The figure shows three views and two pictorial views of one solid part (mm, origin at its lowest corner). Answer the questions. Give positions to 0.01 mm unless a question says otherwise; leave off trailing zeros. Write each loop counter-clockwise with the first axis right and the second up, starting at its lowest first coordinate (ties: lowest second). Pieces come first, ordered by that corner, then holes. Notation, with made-up numbers: (15, 24) - (51, 24) arc R23 cw to (51, 44) - close; hole circle Ø11 at (-40, 25). An arc over 180 degrees is marked (long way). Use CSV: the item, a comma, the result in double quotes. Start each with the question number.
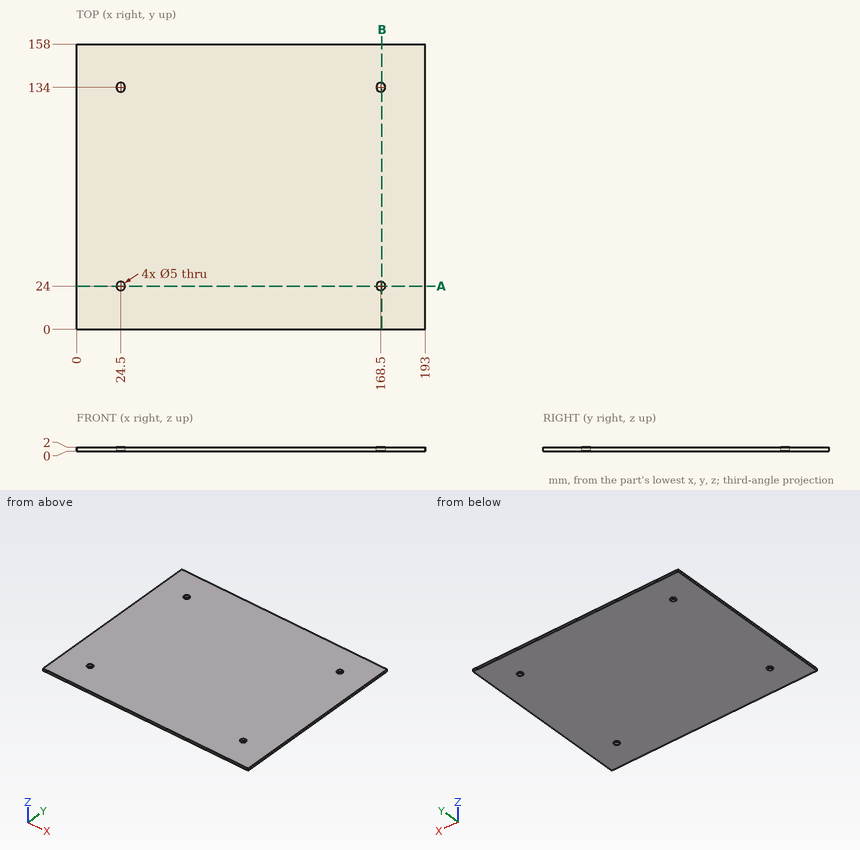
(1) Given P1, Ø8, axis at x = 168.5, y = 24, coming from the +Z side, flat-ended and moving along its own axis, determine where the tip first touches the part or whether it passes through.
(2) The part is cut by section A-A on y = 24. Write down the section's boundary in (x, z), plus the area to 3 significant figures.
(3) The part is cut by section B-B on x = 169. Write down the section's boundary in (y, z).
(4) Consider probe 1 along X at (y, z) = (134, 0.85); probe 2 along Y at (x, z) = (168.5, 1.15). Determine where each line is inside the solid, lowest interval first.
Reported:
1,P1,"z = 2"
2,outline,"(0, 0) - (22, 0) - (22, 2) - (0, 2) - close; (27, 0) - (166, 0) - (166, 2) - (27, 2) - close; (171, 0) - (193, 0) - (193, 2) - (171, 2) - close"
2,area,"366 mm²"
3,outline,"(0, 0) - (21.55, 0) - (21.55, 2) - (0, 2) - close; (26.45, 0) - (131.55, 0) - (131.55, 2) - (26.45, 2) - close; (136.45, 0) - (158, 0) - (158, 2) - (136.45, 2) - close"
4,probe 1,"0 to 22, 27 to 166, 171 to 193"
4,probe 2,"0 to 21.5, 26.5 to 131.5, 136.5 to 158"
